from build123d import *

# Parameters (mm, degrees)
SKETCH_1_W          = 160
SKETCH_1_H          = 109
EXTRUDE_1_DEPTH     = 1.8
SKETCH_2_R          = 2
CUT_EXTRUDE_1_DEPTH = 97.816785735
SKETCH_3_W          = 141
SKETCH_3_H          = 2.15
CUT_EXTRUDE_3_DEPTH = 97.816785735
SKETCH_4_W          = 141
SKETCH_4_H          = 104.7
EXTRUDE_2_DEPTH     = 8.5
SKETCH_5_W          = 122
SKETCH_5_H          = 92
CUT_EXTRUDE_4_DEPTH = 1
SKETCH_6_R          = 0.5
CUT_EXTRUDE_5_DEPTH = 98.172526982
SKETCH_7_W          = 141
SKETCH_7_H          = 104.7
EXTRUDE_3_DEPTH     = 1.7


with BuildPart() as part:
    # 草图1 → 拉伸1 (new body)
    with BuildSketch(Plane(origin=(0, 0, 0), x_dir=(1, 0, 0), z_dir=(0, 1, 0))):
        Rectangle(SKETCH_1_W, SKETCH_1_H)
    extrude(amount=EXTRUDE_1_DEPTH)

    # 草图2 → 切除-拉伸1 (cut, through all)
    with BuildSketch(Plane(origin=(0, 1.8, 0), x_dir=(-1, 0, 0), z_dir=(0, 1, 0))):
        with Locations(Location((-76, -50.5, 0), (0, 0, 90))):
            Circle(SKETCH_2_R)
        with Locations(Location((-76, 50.5, 0), (0, 0, 90))):
            Circle(SKETCH_2_R)
        with Locations(Location((76, 50.5, 0), (0, 0, 90))):
            Circle(SKETCH_2_R)
        with Locations(Location((76, -50.5, 0), (0, 0, 90))):
            Circle(SKETCH_2_R)
    extrude(amount=-CUT_EXTRUDE_1_DEPTH, mode=Mode.SUBTRACT)

    # 草图3 → 切除-拉伸3 (cut, through all)
    with BuildSketch(Plane(origin=(0, 1.8, 0), x_dir=(-1, 0, 0), z_dir=(0, 1, 0))):
        with Locations((-1.5, -53.425)):
            Rectangle(SKETCH_3_W, SKETCH_3_H)
        with Locations((-1.5, 53.425)):
            Rectangle(SKETCH_3_W, SKETCH_3_H)
    extrude(amount=-CUT_EXTRUDE_3_DEPTH, mode=Mode.SUBTRACT)

    # 草图4 → 拉伸2 (add)
    with BuildSketch(Plane(origin=(0, 1.8, 0), x_dir=(-1, 0, 0), z_dir=(0, 1, 0))):
        with Locations((-1.5, 0)):
            Rectangle(SKETCH_4_W, SKETCH_4_H)
    extrude(amount=EXTRUDE_2_DEPTH)

    # 草图5 → 切除-拉伸4 (cut)
    with BuildSketch(Plane(origin=(0, 10.3, 0), x_dir=(-1, 0, 0), z_dir=(0, 1, 0))):
        with Locations((-6, 0)):
            Rectangle(SKETCH_5_W, SKETCH_5_H)
    extrude(amount=-CUT_EXTRUDE_4_DEPTH, mode=Mode.SUBTRACT)

    # 草图6 → 切除-拉伸5 (cut, through all)
    with BuildSketch(Plane(origin=(0, 1.8, 0), x_dir=(-1, 0, 0), z_dir=(0, 1, 0))):
        with Locations(Location((78.72, 17.5, 0), (0, 0, 90))):
            Circle(SKETCH_6_R)
        with Locations(Location((78.72, 14.96, 0), (0, 0, 90))):
            Circle(SKETCH_6_R)
        with Locations(Location((78.72, 12.42, 0), (0, 0, 90))):
            Circle(SKETCH_6_R)
        with Locations(Location((78.72, 9.88, 0), (0, 0, 90))):
            Circle(SKETCH_6_R)
        with Locations(Location((78.72, 7.34, 0), (0, 0, 90))):
            Circle(SKETCH_6_R)
        with Locations(Location((78.72, 4.8, 0), (0, 0, 90))):
            Circle(SKETCH_6_R)
        with Locations(Location((78.72, 2.26, 0), (0, 0, 90))):
            Circle(SKETCH_6_R)
        with Locations(Location((78.72, -0.28, 0), (0, 0, 90))):
            Circle(SKETCH_6_R)
        with Locations(Location((78.72, -2.82, 0), (0, 0, 90))):
            Circle(SKETCH_6_R)
        with Locations(Location((78.72, -5.36, 0), (0, 0, 90))):
            Circle(SKETCH_6_R)
        with Locations(Location((78.72, -7.9, 0), (0, 0, 90))):
            Circle(SKETCH_6_R)
        with Locations(Location((78.72, -10.44, 0), (0, 0, 90))):
            Circle(SKETCH_6_R)
        with Locations(Location((78.72, -12.98, 0), (0, 0, 90))):
            Circle(SKETCH_6_R)
        with Locations(Location((78.72, -15.52, 0), (0, 0, 90))):
            Circle(SKETCH_6_R)
        with Locations(Location((78.72, -18.06, 0), (0, 0, 90))):
            Circle(SKETCH_6_R)
        with Locations(Location((78.72, -20.6, 0), (0, 0, 90))):
            Circle(SKETCH_6_R)
        with Locations(Location((78.72, -23.14, 0), (0, 0, 90))):
            Circle(SKETCH_6_R)
        with Locations(Location((78.72, -25.68, 0), (0, 0, 90))):
            Circle(SKETCH_6_R)
        with Locations(Location((78.72, -28.22, 0), (0, 0, 90))):
            Circle(SKETCH_6_R)
        with Locations(Location((78.72, -30.76, 0), (0, 0, 90))):
            Circle(SKETCH_6_R)
    extrude(amount=-CUT_EXTRUDE_5_DEPTH, mode=Mode.SUBTRACT)

    # 草图7 → 拉伸3 (add)
    with BuildSketch(Plane.XZ):
        with Locations((1.5, 0)):
            Rectangle(SKETCH_7_W, SKETCH_7_H)
    extrude(amount=EXTRUDE_3_DEPTH)


solid = part.part
Work out the finished part from the listing and answer in its coordinate system (mm). A direction names the side the tool comes from. Coordinates: 2 decimals unless noted, no trailing zeros. Order: outer loops, then holes, each group sorted by start corner. A loop starts at its lowest first (then second) coordinate and runs counter-clockwise, first axis right, second up. Notation, with made-up numbers: (-30, 36.5) - (7, 36.5) arc R29 cw to (7, 70.5) - close; hole circle Ø10 at (-2, 16.5). An arc over 180 degrees is marked (long way). Put each result on its own line as item: value. Start each with the question number.
1) Find section B-B (x = -8). Give the vertices of the cut face in (y, z), plus the area to 3 significant figures.
2) Find the intervals of material crossed by line 1 (X direction, y = 0.8, z = -5.36); line 2 (Z direction, x = 26, y = 9.75); line 3 (X direction, y = 1.2, z = -50.5), in increasing order. Write a range as from..to.
3) For faces 1 (the flat face through (76, 0, -1)), 2 (the flat face through (-75, 1.8, -1)), 3 (the flat face through (1, 4, 52.35)), determine the directions among +Z, -Z, +X, -X, +Y, -Y from which every point of the face is accessible in a straight line to the end or side of a thin tool.
4) Find section C-C (y = 4). Give the vertices of the cut face in (x, z), plus the area to 3 significant figures.
5) Flat-ended cylindrical pins translate along their axes: pin 1 (0.8 mm diameter, centred on x = -19.5, y = 10, fed in from +Z); pin 2 (0.8 mm diameter, centred on y = 10, z = -12, fed in from +X); pin 3 (4.5 mm diameter, centred on x = -76, z = -50.5, fed in from +Y). Find the tip coordinate at first contact, or state that the pin passes through.
6) Find section A-A (z = -50.5). Give the vertices of the cut face in (x, y), plus the area to 3 significant figures.
Results list:
1. outline: (-1.7, -52.35) - (10.3, -52.35) - (10.3, -46) - (9.3, -46) - (9.3, 46) - (10.3, 46) - (10.3, 52.35) - (-1.7, 52.35) - close
1. area: 1,160 mm^2
2. line 1: x = -80..-79.22, -78.22..80
2. line 2: z = -52.35..-46, 46..52.35
2. line 3: x = -80..-78, -74..74, 78..80
3. face 1: +Z, -Z, +X, -Y
3. face 2: +Z, -Z, -X, +Y
3. face 3: +Z, +Y, -Y
4. outline: (-69, -52.35) - (72, -52.35) - (72, 52.35) - (-69, 52.35) - close
4. area: 14,800 mm^2
5. pin 1: stops at z = 52.35
5. pin 2: stops at x = 72
5. pin 3: stops at y = 1.8
6. outline: (-80, 0) - (-78, 0) - (-78, 1.8) - (-80, 1.8) - close; (-74, 0) - (-69, 0) - (-69, -1.7) - (72, -1.7) - (72, 0) - (74, 0) - (74, 1.8) - (72, 1.8) - (72, 10.3) - (-69, 10.3) - (-69, 1.8) - (-74, 1.8) - close; (78, 0) - (80, 0) - (80, 1.8) - (78, 1.8) - close
6. area: 1,710 mm^2
